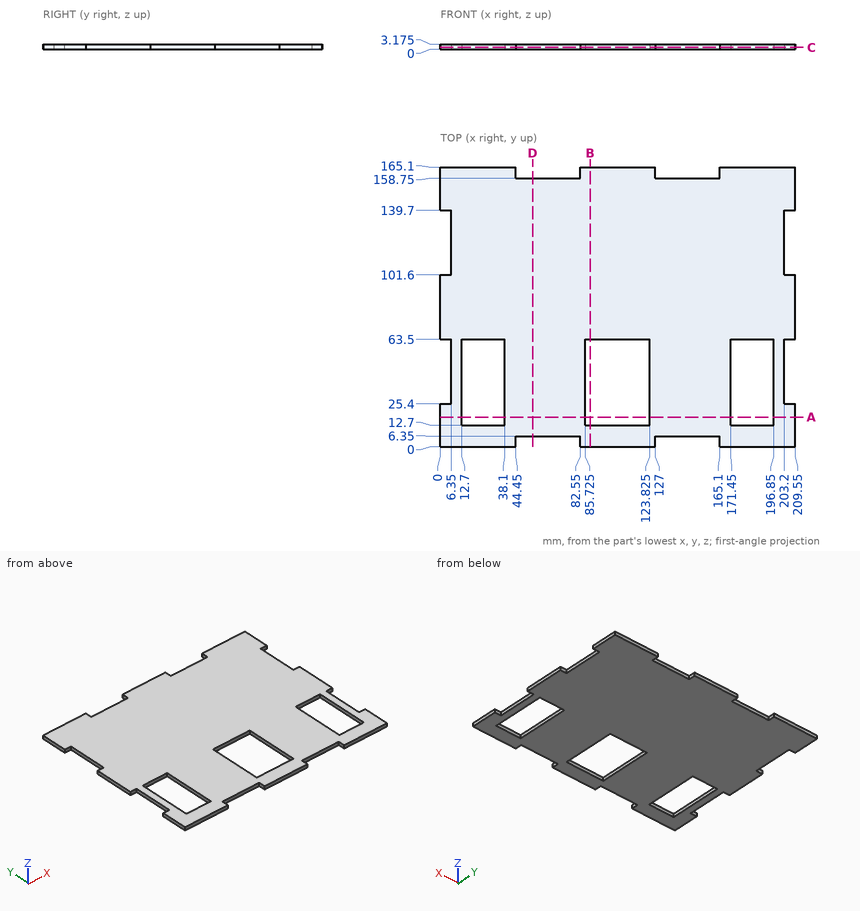
Source: three-view drawing plus pictorial views. Frame: mm from the lowest corner of the part. Coordinates: 2 decimals unless noted, no trailing zeros. Loops run counter-clockwise (first coordinate to the right, second up) from the corner with the lowest first, then second, coordinate; pieces in that order, holes last. Notation, with made-up numbers: (31, 23.5) - (38, 23.5) arc R14 ccw to (38, 40.5) - close; hole circle Ø8 at (70.25, 3). An arc over 180 degrees is marked (long way). One line per question, with ' | ' between items.
1) Section D-D, the plane x = 54.5. Return loops of the section in (y, z) (3 decimals), then the cut area to 3 significant figures.
Report:
outline: (6.35, 0) - (158.75, 0) - (158.75, 3.175) - (6.35, 3.175) - close | area: 484 mm²
2) Section A-A, the plane y = 17.5. Return loops of the section in (x, z) (3 decimals).
Report:
outline: (0, 0) - (12.7, 0) - (12.7, 3.175) - (0, 3.175) - close; (38.1, 0) - (85.725, 0) - (85.725, 3.175) - (38.1, 3.175) - close; (123.825, 0) - (171.45, 0) - (171.45, 3.175) - (123.825, 3.175) - close; (196.85, 0) - (209.55, 0) - (209.55, 3.175) - (196.85, 3.175) - close
3) Section C-C, the plane z = 1.15. Give the number of separate pieces and of enclosed holes in the cut face, then the cut area to 3 significant figures.
Report:
separate pieces: 1 | enclosed holes: 3 | area: 28,100 mm²
4) First-contact query: P1, Ø1, axis at y = 40, z = 2, coming from the +X side; P2, Ø1, axis at x = 2, z = 1, coming from the -Y side; P3, Ø1, axis at y = 28.5, z = 2, coming from the -X side; P4, Ø1, axis at x = 67.5, z = 1, coming from the +Y side. Flat tips, straight axial feed; report the tip coordinate or a pass-through.
Report:
P1: stops at x = 203.2 | P2: stops at y = 0 | P3: stops at x = 6.35 | P4: stops at y = 158.75
5) Line query: line 1 along X through (y, z) = (25.5, 1.25) (3 decimals); line 2 along Y through (x, z) = (87.5, 1.5); line 3 along X through (y, z) = (128, 0.95). Output: solid intervals per line, ascending.
Report:
line 1: x = 6.35 to 12.7, 38.1 to 85.725, 123.825 to 171.45, 196.85 to 203.2 | line 2: y = 0 to 12.7, 63.5 to 165.1 | line 3: x = 6.35 to 203.2
6) Section B-B, the plane x = 88.5. Return loops of the section in (y, z) (3 decimals).
Report:
outline: (0, 0) - (12.7, 0) - (12.7, 3.175) - (0, 3.175) - close; (63.5, 0) - (165.1, 0) - (165.1, 3.175) - (63.5, 3.175) - close
